Design review of the part built by this model. Coordinates are the model's own, in mm. A direction names the side the tool comes from. Coordinates: 2 decimals unless noted, no trailing zeros. Order: outer loops, then holes, each group sorted by start corner. A loop starts at its lowest first (then second) coordinate and runs counter-clockwise, first axis right, second up.
from build123d import *

# Parameters (mm, degrees)
BOSS_EXTRUDE1_DEPTH = 1.5875


with BuildPart() as part:
    # Sketch1 → Boss-Extrude1 (new body)
    with BuildSketch(Plane.XY):
        with BuildLine():
            Line((0, 0), (0, 3.175))
            ThreePointArc((0, 3.175), (0.79375, 3.96875), (1.5875, 3.175))
            Line((1.5875, 3.175), (1.5875, 0))
            Line((1.5875, 0), (69.9135, 15.774300027))
            Line((69.9135, 15.774300027), (69.9135, 19.146896146))
            ThreePointArc((69.9135, 19.146896146), (70.619414052, 20.019686772), (71.492204678, 19.31377272))
            Line((71.492204678, 19.31377272), (71.492204678, 16.13877272))
            Line((71.492204678, 16.13877272), (74.631909532, 16.8636307))
            Line((74.631909532, 16.8636307), (73.203470337, 23.050880612))
            Line((73.203470337, 23.050880612), (1.5875, 6.517031084))
            Line((1.5875, 6.517031084), (-3.518428564, 5.338234593))
            Line((-3.518428564, 5.338234593), (-2.286, 0))
            Line((-2.286, 0), (0, 0))
        make_face()
    extrude(amount=BOSS_EXTRUDE1_DEPTH)


solid = part.part
1. To check wall thickness, follow line 1 (Y direction, x = 54, z = 1.4); line 2 (Y direction, x = 26, z = 0.4). State the ranges of each line that lie inside material, in increasing order.
2. Mouldability with a two-part tool opening along X and no side actions: class faces 3 (the flat face through (35, 10, 1.588)), 4 (the flat face through (73.93, 19.91, 0.78)), 5 (the flat face through (-2.91, 2.71, 0.78)), 6 (the flat face through (69.914, 17, 1)) as pulls with the +X half, pulls with the -X half, needs draft (parallel to the pull), parting line crosses it, or undercut.
3. Add section B-B (y = 2.5). Give the boundary of the cut face in (x, z), and give its area (3 significant figures).
4. For faces 1 (the flat face through (35, 10, 0)), 2 (the flat face through (0, 2, 1)), list the 3-axis set-ups (+Z, -Z, +X, -X, +Y, -Y) from which the entire face can be reached by the end or side of a thin tool; tool diameter is ignored.
5. Add section A-A (z = 1.3). Give the boundary of the cut face in (x, y) (1 decimal).
6. Add section C-C (x = 10). Give the boundary of the cut face in (y, z).
7. Insertion check: pin 1 (0.5 mm diameter, centred on y = 18, z = 1, fed in from +X). The pin has a flat end and moves straight along its axis. Give the tip position at first contact, or say it passes through.
Solution:
1. line 1: y = 12.1 to 18.62
1. line 2: y = 5.64 to 12.15
2. face 3: needs draft
2. face 4: pulls with the +X half
2. face 5: pulls with the -X half
2. face 6: undercut
3. outline: (-2.86, 0) - (0, 0) - (0, 1.59) - (-2.86, 1.59) - close; (1.59, 0) - (12.42, 0) - (12.42, 1.59) - (1.59, 1.59) - close
3. area: 21.7 mm2
4. face 1: -Z, +X, -X, +Y, -Y
4. face 2: +Z, -Z, -Y
5. outline: (-3.5, 5.3) - (-2.3, 0) - (0, 0) - (0, 3.2) arc R0.8 cw to (1.6, 3.2) - (1.6, 0) - (69.9, 15.8) - (69.9, 19.1) arc R0.8 cw to (71.5, 19.3) - (71.5, 16.1) - (74.6, 16.9) - (73.2, 23.1) - close
6. outline: (1.94, 0) - (8.46, 0) - (8.46, 1.59) - (1.94, 1.59) - close
7. pin 1: stops at x = 74.43
